Could you check a few things on this drawing? It's one solid part, dimensions in mm from its lowest x, y, z. A direction names the side the tool comes from. Coordinates: 2 decimals unless noted, no trailing zeros. Loops run counter-clockwise (first coordinate to the right, second up) from the corner with the lowest first, then second, coordinate; pieces in that order, holes last. Notation, with made-up numbers: (-10.5, 87) -> (12.5, 87) arc R15 ccw to (12.5, 109) -> close; hole circle Ø11 at (29.5, 89). An arc over 180 degrees is marked (long way). One line per question, with ' | ' between items. Start each with the question number.
(1) If we mould it in two halves opening along X, with no side actions, what happens to the marked faces 3, 4 and 5? For each: pulls with the +X half, pulls with the -X half, needs draft (parallel to the pull), parting line crosses it, or undercut.
(2) Which directions (+Z, -Z, +X, -X, +Y, -Y) give clear straight access to the entire face, cutting with the end or side of a thin tool? Please do the marked faces 1 and 2.
(3) Suppose I cut it at A-A (x = 45). Please give me the cut outline in (y, z).
(4) Suppose I cut it at B-B (y = 36). Please give me the cut outline in (x, z).
(5) If I drill on line 1 along Y through (x, z) = (3, 4.75); line 2 along X through (y, z) = (4, 5); line 3 along Y through (x, z) = (65, 6.75), over which ranges is the centre line in solid material (lowest first)?
(6) Suppose I cut it at D-D (x = 3). Please give me the cut outline in (y, z).
(7) I'm going to push flat-ended pins straight in: pin 1 Ø2 at (x, z) = (78, 8.5) entering from -Y; pin 2 Ø2.5 at (x, y) = (97, 4) entering from -Z; pin 3 Ø1.5 at (y, z) = (27.5, 8.5) entering from -X; pin 4 Ø1.5 at (x, z) = (50, 10.5) entering from +Y. Where does each tip first touch, or does it pass through?
(8) Suppose I cut it at C-C (z = 8.5). Please give me the cut outline in (x, y), plus the area to 3 significant figures.
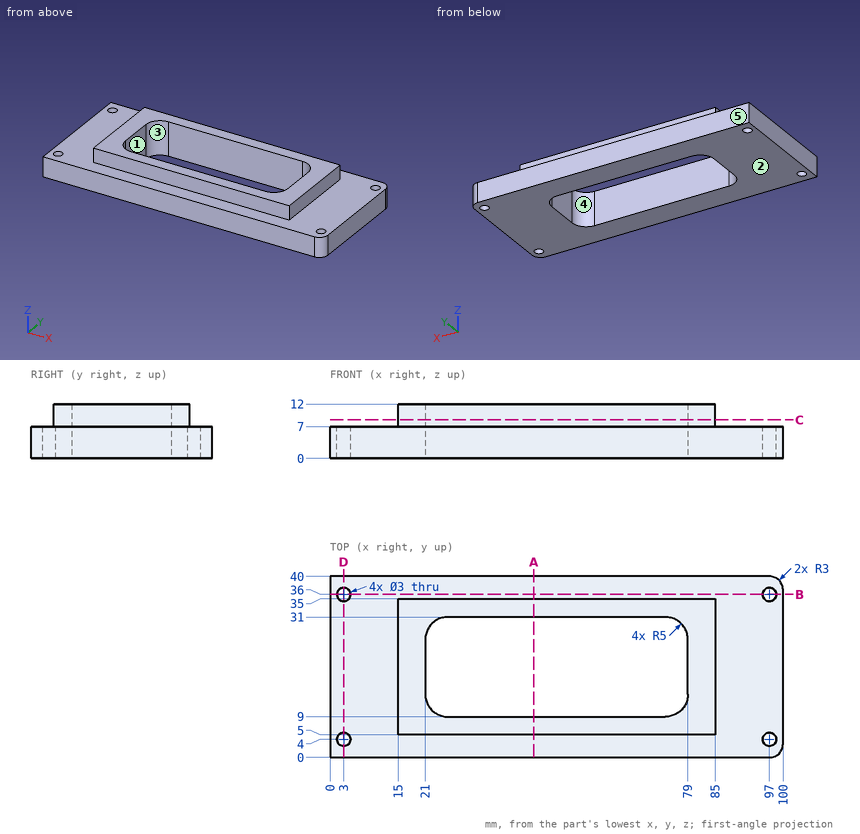
Checks:
1) face 3: undercut | face 4: undercut | face 5: needs draft
2) face 1: +Z, -Z | face 2: -Z, +X, -X, +Y, -Y
3) outline: (0, 0) -> (9, 0) -> (9, 12) -> (5, 12) -> (5, 7) -> (0, 7) -> close; (31, 0) -> (40, 0) -> (40, 7) -> (35, 7) -> (35, 12) -> (31, 12) -> close
4) outline: (0, 0) -> (1.5, 0) -> (1.5, 7) -> (0, 7) -> close; (4.5, 0) -> (95.5, 0) -> (95.5, 7) -> (4.5, 7) -> close; (98.5, 0) -> (100, 0) -> (100, 7) -> (98.5, 7) -> close
5) line 1: y = 0 to 2.5, 5.5 to 34.5, 37.5 to 40 | line 2: x = 0 to 1.5, 4.5 to 95.5, 98.5 to 100 | line 3: y = 0 to 9, 31 to 40
6) outline: (0, 0) -> (2.5, 0) -> (2.5, 7) -> (0, 7) -> close; (5.5, 0) -> (34.5, 0) -> (34.5, 7) -> (5.5, 7) -> close; (37.5, 0) -> (40, 0) -> (40, 7) -> (37.5, 7) -> close
7) pin 1: stops at y = 5 | pin 2: passes through | pin 3: stops at x = 15 | pin 4: stops at y = 35
8) outline: (15, 5) -> (85, 5) -> (85, 35) -> (15, 35) -> close; hole (21, 14) arc R5 ccw to (26, 9) -> (74, 9) arc R5 ccw to (79, 14) -> (79, 26) arc R5 ccw to (74, 31) -> (26, 31) arc R5 ccw to (21, 26) -> close | area: 845 mm^2
